```python
from build123d import *

# Parameters (mm, degrees)
F0_W     = 100
F0_H     = 350
F0_R     = 10
F1_DEPTH = 10
F2_DEPTH = 20
F3_R     = 1.5
F4_DEPTH = 20
F5_R     = 1


with BuildPart() as f1:
    # F0 (on Front) → F1 (new body)
    with BuildSketch(Plane.XZ):
        with Locations((0, -100)):
            Rectangle(F0_W, F0_H)
        with Locations((-30, 0)):
            Circle(F0_R, mode=Mode.SUBTRACT)
        with Locations((30, 0)):
            Circle(F0_R, mode=Mode.SUBTRACT)
    extrude(amount=F1_DEPTH)

    # F0 (on Front) → F2 (join)
    with BuildSketch(Plane.XZ):
        with Locations((-30, 0)):
            Circle(F0_R)
        with Locations((30, 0)):
            Circle(F0_R)
    extrude(amount=F2_DEPTH)

    # F3 (on face) → F4 (join)
    with BuildSketch(Plane.XZ.offset(10)):
        with Locations((-25, -100)):
            Circle(F3_R)
    extrude(amount=F4_DEPTH)

    # F5
    f5_edges = [f1.edges().sort_by_distance(p)[0] for p in [
        (-26.5, -30, -100),
    ]]
    fillet(f5_edges, radius=F5_R)


solid = f1.part
```
Part model, mm, in its own coordinate system. A direction names the side the tool comes from. Round coordinates to 2 decimals unless told otherwise and drop trailing zeros. Loops run counter-clockwise (first coordinate to the right, second up) from the corner with the lowest first, then second, coordinate; pieces in that order, holes last.
1. Flat gauge pins, fed straight in: pin 1 (8 mm diameter, centred on y = -23.5, z = 5, fed in from +X); pin 2 (22 mm diameter, centred on x = 28.5, z = -2.5, fed in from -Y); pin 3 (12 mm diameter, centred on x = 16.5, y = -26.5, fed in from -Z); pin 4 (4 mm diameter, centred on x = -20.5, z = -130, fed in from -Y). Where does each tip first touch, or does it go through?
Solutions:
pin 1: stops at x = 39.52
pin 2: stops at y = -20
pin 3: passes through
pin 4: stops at y = -10
2. Slice it at A-A (y = -16.5). Give the cut face in (x, z).
Solutions:
outline: circle Ø20 at (-30, 0); circle Ø3 at (-25, -100); circle Ø20 at (30, 0)
3. Slice it at D-D (x = -15). Give the cut face in (y, z), and give its area (3 significant figures).
Solutions:
outline: (-10, -275) - (0, -275) - (0, 75) - (-10, 75) - close
area: 3,500 mm2
4. Slice it at C-C (z = -54.5). Give the cut face in (x, y), and give its area (3 significant figures).
Solutions:
outline: (-50, -10) - (50, -10) - (50, 0) - (-50, 0) - close
area: 1,000 mm2
5. 3-axis set-ups, long thin cutter, end or side, ignore diameter. For faces 1 (the face through (-50, -5, -102)), 2 (the face through (39.54, -14.93, 3)): which of +Z, -Z, +X, -X, +Y, -Y reach the whole face in a straight line?
Solutions:
face 1: +Z, -Z, -X, +Y, -Y
face 2: -Y
6. Two-plate mould, pull along X, no slides. Class faces 3 (the face through (-40, -15, 0)), 4 (the face through (-30, -20, 0)), 5 (the face through (50, -5, -102)): pulls with the +X half, pulls with the -X half, needs draft (parallel to the pull), parting line crosses it, or undercut.
Solutions:
face 3: undercut
face 4: needs draft
face 5: pulls with the +X half
7. Slice it at B-B (x = 30). Give the cut face in (y, z).
Solutions:
outline: (-20, -10) - (-10, -10) - (-10, -275) - (0, -275) - (0, 75) - (-10, 75) - (-10, 10) - (-20, 10) - close
8. Drill centre line: line 1 along Y through (x, z) = (38.5, -23.5). Where is it in solid material? Low to high.
Solutions:
line 1: y = -10 to 0
